Build history of the part. All positions in model axes, mm. Coordinates: 2 decimals unless noted, no trailing zeros. Loops run counter-clockwise (first coordinate to the right, second up) from the corner with the lowest first, then second, coordinate; pieces in that order, holes last.
(1) Slice it at A-A (x = -17). Give the cut face in (y, z), and give its area (3 significant figures).
(2) Two-plate mould, pull along X, no slides. Class faces 1 (the face through (-31.217, 8.098, 1.486)), 2 (the face through (-56, -1, 3)), 3 (the face through (-57.97, 0.74, 2.75)): pulls with the +X half, pulls with the -X half, needs draft (parallel to the pull), parting line crosses it, or undercut.
(3) Wall check: L1, parallel to Y at x = -17, z = 1.9; L2, parallel to Y at x = -74, z = 0.6; L3, parallel to X at y = -15.5, z = 0.7. Give the ranges that are in metal, low to high.
(4) Flat gauge pins, fed straight in: P1, Ø1, axis at x = -63.5, z = 0.5, coming from the -Y side; P2, Ø1, axis at y = 3, z = 2, coming from the +X side; P3, Ø1, axis at y = 1, z = 2.5, coming from the +X side. Where does each tip first touch, or does it go through?
from build123d import *

# Parameters (mm, degrees)
SKETCH1_R             = 3
SKETCH1_R_2           = 1.5
BOSS_EXTRUDE1_DEPTH   = 3
BOSS_EXTRUDE1_2_DEPTH = 3
EXTRUDE_THIN1_DEPTH   = 3
FILLET1_R             = 5
CHAMFER1_SIZE         = 0.5


with BuildPart() as part:
    # Sketch1 → Boss-Extrude1 (new body)
    with BuildSketch(Plane.XY):
        with Locations((-83.950540957, -19.912145865)):
            Circle(SKETCH1_R)
        with Locations((-83.950540957, -19.912145865)):
            Circle(SKETCH1_R_2, mode=Mode.SUBTRACT)
    extrude(amount=BOSS_EXTRUDE1_DEPTH)



with BuildPart() as body_2:
    # Sketch1 → Boss-Extrude1 2 (new body)
    with BuildSketch(Plane.XY):
        with Locations((-17, 9.92820323)):
            Circle(SKETCH1_R)
        with Locations((-17, 9.92820323)):
            Circle(SKETCH1_R_2, mode=Mode.SUBTRACT)
    extrude(amount=BOSS_EXTRUDE1_2_DEPTH)


with BuildPart() as part_1:
    add(part.part)

    add(body_2.part)  # Extrude-Thin1 merges body 2
    # Sketch2 → Extrude-Thin1 (add)
    with BuildSketch(Plane.XY):
        with BuildLine():
            ThreePointArc((-81.866086482, -18.096227729), (-76.0782564, -7.689979577), (-65.226210809, -2.788746653))
            Line((-65.226210809, -2.788746653), (-50.342422521, -1.224397467))
            ThreePointArc((-50.342422521, -1.224397467), (-43.92427654, 0.448702034), (-38.289233854, 3.947009295))
            ThreePointArc((-38.289233854, 3.947009295), (-29.303097517, 8.716235486), (-19.143567587, 9.245495681))
            Line((-19.143567587, 9.245495681), (-18.648168411, 12.204309575))
            ThreePointArc((-18.648168411, 12.204309575), (-30.10325921, 11.607557202), (-40.235323233, 6.230151019))
            ThreePointArc((-40.235323233, 6.230151019), (-45.107146333, 3.205660332), (-50.65600791, 1.759168219))
            Line((-50.65600791, 1.759168219), (-65.539796199, 0.194819033))
            ThreePointArc((-65.539796199, 0.194819033), (-78.10933943, -5.482106907), (-84.813179718, -17.535298624))
            Line((-84.813179718, -17.535298624), (-81.866086482, -18.096227729))
        make_face()
    extrude(amount=EXTRUDE_THIN1_DEPTH)

    # Fillet1
    fillet1_edges = [part_1.edges().sort_by_distance(p)[0] for p in [
        (-84.706300556, -17.008901571, 1.5),
        (-81.809477217, -17.810754407, 1.5),
        (-18.904716374, 12.245972748, 1.5),
        (-19.94680617, 9.365767994, 1.5),
    ]]
    fillet(fillet1_edges, radius=FILLET1_R)

    # Chamfer1
    chamfer1_edges = [part_1.edges().sort_by_distance(p)[0] for p in [
        (-77.195374918, -4.686748809, 0),
        (-75.062303692, -6.819526639, 3),
        (-57.784316665, -2.00657206, 3),
        (-43.92427654, 0.448702034, 3),
        (-45.107146333, 3.205660332, 0),
        (-58.097902055, 0.976993626, 0),
        (-45.107146333, 3.205660332, 3),
        (-58.097902055, 0.976993626, 3),
        (-77.195374918, -4.686748809, 3),
        (-75.062303692, -6.819526639, 0),
        (-43.92427654, 0.448702034, 0),
        (-57.784316665, -2.00657206, 0),
        (-84.737508384, -22.807086671, 0),
        (-84.737508384, -22.807086671, 3),
        (-31.106705209, 8.137983689, 0),
        (-31.106705209, 8.137983689, 3),
        (-14.083717416, 9.224430618, 0),
        (-14.083717416, 9.224430618, 3),
        (-30.92519874, 11.365731626, 0),
        (-30.92519874, 11.365731626, 3),
        (-84.860623121, -16.505866782, 3),
        (-84.860623121, -16.505866782, 0),
        (-81.450241332, -17.19340927, 3),
        (-81.450241332, -17.19340927, 0),
        (-20.896879636, 9.132244106, 3),
        (-20.896879636, 9.132244106, 0),
        (-19.18823543, 12.449634759, 3),
        (-19.18823543, 12.449634759, 0),
    ]]
    chamfer(chamfer1_edges, length=CHAMFER1_SIZE)


solid = part_1.part
Response values:
1. outline: (6.93, 0.5) - (7.43, 0) - (8.43, 0) - (8.43, 3) - (7.43, 3) - (6.93, 2.5) - close; (11.43, 0) - (12.43, 0) - (12.93, 0.5) - (12.93, 2.5) - (12.43, 3) - (11.43, 3) - close
1. area: 8.50 mm2
2. face 1: undercut
2. face 2: needs draft
2. face 3: pulls with the -X half
3. L1: y = 6.93 to 8.43, 11.43 to 12.93
3. L2: y = -6.03 to -2.5
3. L3: x = -84.34 to -81.18
4. P1: stops at y = -2.66
4. P2: stops at x = -38.83
4. P3: stops at x = -41.8
